```python
from build123d import *

# Parameters (mm, degrees)
F0_W      = 18.5
F0_H      = 26
F1_DEPTH  = 1.5
F2_W      = 12.1
F2_H      = 12.1
F3_DEPTH  = 5
F4_R      = 3.5
F5_DEPTH  = 21.5
F7_DEPTH  = 10.7
F8_R      = 6
F9_DEPTH  = 15
F10_DEPTH = 25


with BuildPart() as f1:
    # F0 (on Top) → F1 (new body)
    with BuildSketch(Plane.XY):
        Rectangle(F0_W, F0_H)
    extrude(amount=F1_DEPTH)

    # F2 (on face) → F3 (join)
    with BuildSketch(Plane.XY.offset(1.5)):
        with Locations((0, 5.640632961)):
            Rectangle(F2_W, F2_H)
    extrude(amount=F3_DEPTH)

    # F4 (on face) → F5 (join)
    with BuildSketch(Plane.XY.offset(6.5)):
        with Locations((0, 5.640632961)):
            Circle(F4_R)
    extrude(amount=F5_DEPTH)

    # F6 (on face) → F7 (cut)
    with BuildSketch(Plane.XY.offset(28)):
        with BuildLine():
            Line((-3.3541019662, 6.640632961), (0, 6.640632961))
            Line((0, 6.640632961), (3.3541019662, 6.640632961))
            ThreePointArc((3.3541019662, 6.640632961), (0, 9.140632961), (-3.3541019662, 6.640632961))
        make_face()
    extrude(amount=-F7_DEPTH, mode=Mode.SUBTRACT)

    # F8 (on face) → F9 (join)
    with BuildSketch(Plane.XY.offset(28)):
        with Locations((0, 5.640632961)):
            Circle(F8_R)
    extrude(amount=F9_DEPTH)

    # F10 (cut): a face of the model
    f10_faces = [f1.faces().sort_by_distance(p)[0] for p in [
        (0, 7.6794032986, 17.3),
    ]]
    extrude(f10_faces, amount=F10_DEPTH, mode=Mode.SUBTRACT)


solid = f1.part
```
Can you work these out from the model? Positions are in its coordinate system, mm. A direction names the side the tool comes from. Give positions to 0.01 mm unless a question says otherwise; leave off trailing zeros. Order: outer loops, then holes, each group sorted by start corner. A loop starts at its lowest first (then second) coordinate and runs counter-clockwise, first axis right, second up. Notation, with made-up numbers: (18.5, 23) - (73.5, 23) arc R22 cw to (73.5, 56) - close; hole circle Ø6 at (12, 33). An arc over 180 degrees is marked (long way). Use a Markdown table: item, result. Add a question column.
Q1. I'm going to push flat-ended pins straight in: pin 1 (1 mm diameter, centred on y = 0.5, z = 35.5, fed in from -X); pin 2 (10 mm diameter, centred on y = 4.5, z = 33, fed in from +X); pin 3 (1.2 mm diameter, centred on x = -1, y = 7.5, fed in from -Z); pin 4 (1.5 mm diameter, centred on y = 2, z = 35.5, fed in from -X). Where does each tip first touch, or does it pass through?
Q2. If we section it at D-D on y = -2.25: Write out the boundary of the cut face in (x, z).
Q3. If we mould it in two halves opening along X, with no side actions, what happens to faces 5 (the flat face through (0, 13, 1)), 6 (the flat face through (-6.05, 6, 4)), 7 (the flat face through (0, 6.641, 30))? For each: released by +X, released by -X, zero draft, split by the parting line, or undercut.
Q4. If we section it at C-C on x = 0: Write out the boundary of the cut face in (y, z), plus the area to 4 significant figures.
Q5. If we section it at A-A on y = 1.25: Write out the boundary of the cut face in (x, z).
Q6. On a 3-axis mill with a long thin cutter (end or side, diameter ignored), from which of +Z, -Z, +X, -X, +Y, -Y can I reach the whole of each face in a straight line? I mean faces 1 (the cylindrical face through (-0.78, 11.59, 35.39)), 2 (the flat face through (0, -0.409, 4)), 3 (the flat face through (6.05, 6, 4)), 4 (the flat face through (3, 3, 28)). Say none if no direction works.
Q7. Please list where these lines run through material, in increasing order: line 1 along Z through (x, y) = (-4, 6); line 2 along Z through (x, y) = (-2.25, 7); line 3 along Y through (x, z) = (-0.25, 21.5).
Q8. If we section it at B-B on x = -5: Write out the boundary of the cut face in (y, z).
Answers follow:
| question | item | result |
|---|---|---|
| 1 | pin 1 | stops at x = -3.8 |
| 1 | pin 2 | stops at x = 6 |
| 1 | pin 3 | stops at z = 0 |
| 1 | pin 4 | stops at x = -5.26 |
| 2 | outline | (-9.25, 0) - (9.25, 0) - (9.25, 1.5) - (-9.25, 1.5) - close |
| 3 | face 5 | zero draft |
| 3 | face 6 | released by -X |
| 3 | face 7 | undercut |
| 4 | outline | (-13, 0) - (13, 0) - (13, 1.5) - (11.69, 1.5) - (11.69, 6.5) - (9.14, 6.5) - (9.14, 17.3) - (6.64, 17.3) - (6.64, 42.3) - (9.14, 42.3) - (9.14, 28) - (11.64, 28) - (11.64, 43) - (-0.36, 43) - (-0.36, 28) - (2.14, 28) - (2.14, 6.5) - (-0.41, 6.5) - (-0.41, 1.5) - (-13, 1.5) - close |
| 4 | area | 367.5 mm^2 |
| 5 | outline | (-9.25, 0) - (9.25, 0) - (9.25, 1.5) - (6.05, 1.5) - (6.05, 6.5) - (-6.05, 6.5) - (-6.05, 1.5) - (-9.25, 1.5) - close; (-4.09, 28) - (4.09, 28) - (4.09, 43) - (-4.09, 43) - close |
| 6 | face 1 | +Z |
| 6 | face 2 | +Z, +X, -X, -Y |
| 6 | face 3 | +Z, +X, +Y, -Y |
| 6 | face 4 | none |
| 7 | line 1 | z = 0 to 6.5, 28 to 43 |
| 7 | line 2 | z = 0 to 17.3, 42.3 to 43 |
| 7 | line 3 | y = 2.15 to 6.64 |
| 8 | outline | (-13, 0) - (13, 0) - (13, 1.5) - (11.69, 1.5) - (11.69, 6.5) - (-0.41, 6.5) - (-0.41, 1.5) - (-13, 1.5) - close; (2.32, 28) - (8.96, 28) - (8.96, 43) - (2.32, 43) - close |
